Could you check a few things on this model? Use its own coordinates, in mm. A direction names the side the tool comes from. Coordinates: 2 decimals unless noted, no trailing zeros. Loops run counter-clockwise (first coordinate to the right, second up) from the corner with the lowest first, then second, coordinate; pieces in that order, holes last. Notation, with made-up numbers: (68.5, 27) - (86.5, 27) arc R30 ccw to (86.5, 64) - close; hole circle Ø3 at (58, 3.5). An arc over 180 degrees is marked (long way). One line per question, with ' | ' between items. Start each with the question number.
1. Please list where these lines run through material, in increasing order: L1, parallel to Y at x = -6.25, z = -0.75; L2, parallel to Z at x = -5.25, y = 4; L3, parallel to X at y = 4.5, z = 5.5. Write a range as [from, to].
2. Which directions (+Z, -Z, +X, -X, +Y, -Y) give clear straight access to the entire face, cutting with the end or side of a thin tool? Please do faces 1 (the flat face through (-0.108, 4, 0)), 2 (the flat face through (-3, 4, -5.91)), 3 (the flat face through (-5.608, 4, 0)), 4 (the flat face through (-3, 4, 6.09)).
3. I want a section at A-A, the plane z = -2.5. Write out the boundary of the cut face in (x, y), then the cut area to 3 significant figures.
4. I want a section at B-B, the plane y = 7.5. Write out the boundary of the cut face in (x, z).
5. I'm going to push flat-ended pins straight in: P1, Ø1.6, axis at x = -2.5, y = 2.5, coming from the -Z side; P2, Ø5, axis at x = -6, y = 8.5, coming from the -Z side; P3, Ø1, axis at y = 3, z = -3, coming from the +X side. Where does each tip first touch, or does it pass through?
from build123d import *

# Parameters (mm, degrees)
SKETCH_1_W      = 5.5
SKETCH_1_H      = 12
EXTRUDE_1_DEPTH = 9
EXTRUDE_2_DEPTH = 2
FILLET_1_R      = 1


with BuildPart() as part:
    # Эскиз1 → Бобышка-Вытянуть1 (new body)
    with BuildSketch(Plane(origin=(0, 0, 0), x_dir=(1, 0, 0), z_dir=(0, 1, 0))):
        with Locations((-2.858040201, -0.090452261)):
            Rectangle(SKETCH_1_W, SKETCH_1_H)
    extrude(amount=EXTRUDE_1_DEPTH)

    # Эскиз3 → Бобышка-Вытянуть2 (add)
    with BuildSketch(Plane(origin=(0, 9, 0), x_dir=(1, 0, 0), z_dir=(0, 1, 0))):
        with BuildLine():
            Line((1.641959799, 3.409547739), (1.641959799, -3.590452261))
            ThreePointArc((1.641959799, -3.590452261), (-2.858040201, -8.090452261), (-7.358040201, -3.590452261))
            Line((-7.358040201, -3.590452261), (-7.358040201, 3.409547739))
            ThreePointArc((-7.358040201, 3.409547739), (-2.858040201, 7.909547739), (1.641959799, 3.409547739))
        make_face()
    extrude(amount=EXTRUDE_2_DEPTH)

    # Скругление1
    fillet_1_edges = [part.edges().sort_by_distance(p)[0] for p in [
        (-2.858040201, 11, -7.909547739),
        (-7.358040201, 11, 0.090452261),
        (-2.858040201, 11, 8.090452261),
        (1.641959799, 11, 0.090452261),
    ]]
    fillet(fillet_1_edges, radius=FILLET_1_R)


solid = part.part
Results are:
1) L1: y = [9, 11] | L2: z = [-5.91, 6.09] | L3: x = [-5.61, -0.11]
2) face 1: +Z, -Z, +X, -Y | face 2: -Z, +X, -X, -Y | face 3: +Z, -Z, -X, -Y | face 4: +Z, +X, -X, -Y
3) outline: (-7.36, 9) - (-5.61, 9) - (-5.61, 0) - (-0.11, 0) - (-0.11, 9) - (1.64, 9) - (1.64, 10) arc R1 ccw to (0.64, 11) - (-6.36, 11) arc R1 ccw to (-7.36, 10) - close | area: 67.1 mm2
4) outline: (-5.61, -5.91) - (-0.11, -5.91) - (-0.11, 6.09) - (-5.61, 6.09) - close
5) P1: stops at z = -5.91 | P2: stops at z = -7.86 | P3: stops at x = -0.11
